The listing builds one solid part. Answer for the finished solid, in the listing's coordinates (mm). Give positions to 0.01 mm unless a question says otherwise; leave off trailing zeros. Loops run counter-clockwise (first coordinate to the right, second up) from the corner with the lowest first, then second, coordinate; pieces in that order, holes last.
Item 1: Section A-A, the plane z = 2.5 is taken. Give the vertices of the cut face in (x, y), and give its area (3 significant figures).
Item 2: Section C-C, the plane x = -0.95 is taken. Give the vertices of the cut face in (y, z), and give its area (3 significant figures).
Item 3: Section B-B, the plane y = -0.65 is taken. Give the vertices of the cut face in (x, z), and give its area (3 significant figures).
Item 4: Consider line 1 along X through (y, z) = (0.05, 6); line 2 along Y through (x, z) = (0.3, 1.5); line 3 along Y through (x, z) = (1.2, 12). Determine where each line is inside the solid, lowest interval first.
from build123d import *

# Parameters (mm, degrees)
PAD001_DEPTH            = 14.2
BODY001_PLACEMENT_ANGLE = 180


with BuildPart() as part:
    # Sketch001 → Pad001 (new body)
    with BuildSketch(Plane.XY):
        with BuildLine():
            ThreePointArc((0, 1.45), (-1.45, 0), (0, -1.45))
            Line((0, -1.45), (0, 1.45))
        make_face()
    pad001 = extrude(amount=PAD001_DEPTH)

    # Mirrored: Pad001 across Sketch001 V_Axis
    add(pad001.mirror(Plane(origin=(0, 0, 0), x_dir=(0, 0, 1), z_dir=(1, 0, 0))))


with BuildPart() as part_1:
    # Body001 placement: moved
    add(part.part.rotate(Axis((0, 0, 0), (0, 0, 1)), BODY001_PLACEMENT_ANGLE))


solid = part_1.part
Worked answers:
1. outline: circle Ø2.9 at (0, 0)
1. area: 6.61 mm2
2. outline: (-1.1, 0) - (1.1, 0) - (1.1, 14.2) - (-1.1, 14.2) - close
2. area: 31.1 mm2
3. outline: (-1.3, 0) - (1.3, 0) - (1.3, 14.2) - (-1.3, 14.2) - close
3. area: 36.8 mm2
4. line 1: x = -1.45 to 1.45
4. line 2: y = -1.42 to 1.42
4. line 3: y = -0.81 to 0.81
